Verification items for the finished model (mm, model axes). Face numbers are marked on the shaded views. Give positions to 0.01 mm unless a question says otherwise; leave off trailing zeros. Loops run counter-clockwise (first coordinate to the right, second up) from the corner with the lowest first, then second, coordinate; pieces in that order, holes last. Notation, with made-up numbers: (3.5, 24) - (56.5, 24) arc R21 ccw to (56.5, 31) - close; hole circle Ø6 at (-24.5, 85). An arc over 180 degrees is marked (long way). Use one line per item in the form item = value.
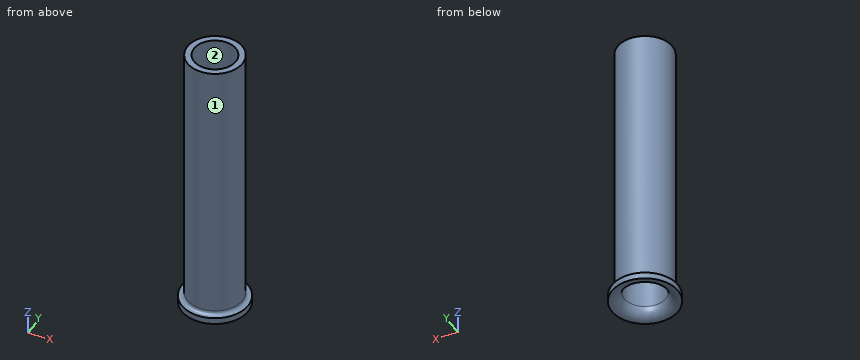
Autodesk Inventor part; units mm, degrees
ref_plane "YZ Plane" through (0, 0, 0) normal (1, 0, 0) x (0, 1, 0)
ref_plane "XZ Plane" through (0, 0, 0) normal (0, 1, 0) x (-1, 0, 0)
ref_plane "XY Plane" through (0, 0, 0) normal (0, 0, 1) x (1, 0, 0)
sketch "Sketch1" plane through (0, 0, 0) normal (0, 0, 1) x (1, 0, 0)
  circle A0 centre (0, 0) radius 13.335
  circle A1 centre (0, 0) radius 10.16
  dimension "d1" = 20.32
  dimension "d5" = 26.67
extrude "Extrusion1" add sketch "Sketch1" along normal blind 58.7375 and the other way blind 71.4375
sketch "Sketch2" plane through (0, 0, 0) normal (0, 1, 0) x (-1, 0, 0)
  line L0 (10.16, -71.4375) -> (10.16, 58.7375) construction
  line L1 (10.16, 58.7375) -> (13.335, 58.7375) construction
  line L2 (13.335, 58.7375) -> (13.335, -71.4375) construction
  line L3 (13.335, -71.4375) -> (10.16, -71.4375)
  line L4 (-10.16, 58.7375) -> (-10.16, -71.4375) construction
  line L5 (-10.16, -71.4375) -> (-13.335, -71.4375) construction
  line L6 (-13.335, -71.4375) -> (-13.335, 58.7375) construction
  line L7 (-13.335, 58.7375) -> (-10.16, 58.7375) construction
  line L8 (13.335, -71.4375) -> (13.335, -73.2656) construction
  line L9 (13.335, -73.2656) -> (16.0701, -73.2656) construction
  spline S0 degree 2 poles (13.335, -71.4375) (13.335, -73.2656) (16.0701, -73.2656) knots 1 1 1 2 2 2
  line L10 (16.0701, -73.2656) -> (16.0701, -76.4406)
  line L11 (0, -105.1255) -> (0, 86.048)
  spline S1 degree 5 poles (10.16, -71.4375) (10.1607, -72.3811) (10.3553, -73.3253) (10.8096, -74.2133) (12.0296, -75.5264) (13.675, -76.2036) (14.4712, -76.3698) (15.2694, -76.4406) (16.0701, -76.4406) knots 0 0 0 0 0 0 0.54113 0.54113 0.54113 1 1 1 1 1 1
  point P0 (0, 0)
revolve "Revolution1" add sketch "Sketch2" angle 360 about axis through (0, 0, -10) along (0, 0, 1)
properties part number "pipe" material "PVC-Piping"
1. Draft check along Y on the marked faces 1 and 2. Enter one of: released by +Y, released by -Y, zero draft, split by the parting line, or undercut.
Result set:
face_1 = split by the parting line
face_2 = undercut
2. Section check A-A, the plane z = 47.5. Record the cut outline in (x, y) (3 decimals).
Result set:
outline = circle Ø26.67 at (0, 0); hole circle Ø20.32 at (0, 0)
3. Scan lines: probe 1 along Y at (x, z) = (0, -33) (3 decimals); probe 2 along X at (y, z) = (-2.5, -58). Record each from-to range of solid material in increasing order.
Result set:
probe_1 = -13.335 to -10.16, 10.16 to 13.335
probe_2 = -13.1 to -9.85, 9.85 to 13.1
4. Depth check by flat-ended pin: pin 1 Ø10 at (x, z) = (-6, 10.5) entering from +Y; pin 2 Ø12 at (x, z) = (9, -23) entering from -Y; pin 3 Ø2 at (x, y) = (-1, 12.5) entering from -Z. Enter the tip coordinate at first touch or a pass-through.
Result set:
pin_1 = 13.3
pin_2 = -12.99
pin_3 = -76.07
